Read the model definition and answer for the solid it produces. Units are mm, in the model's axes. Face numbers are marked on the shaded views. A direction names the side the tool comes from. Round coordinates to 2 decimals unless told otherwise and drop trailing zeros. Order: outer loops, then holes, each group sorted by start corner. A loop starts at its lowest first (then second) coordinate and runs counter-clockwise, first axis right, second up. Notation, with made-up numbers: M -35.75,26.25 L 20.25,26.25 A26 cw 20.25,57.25 Z; hole C 85.5,51.5 d7. An arc over 180 degrees is marked long. Answer as CSV lines item,"result".
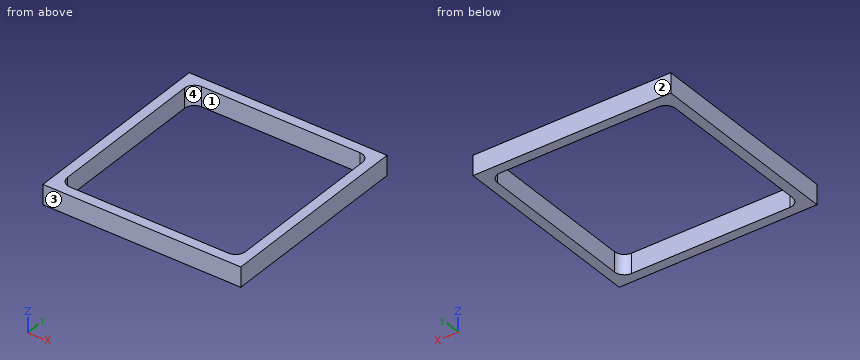
```python
from build123d import *

# Parameters (mm, degrees)
SKETCH1_W           = 127
SKETCH1_H           = 127
SKETCH1_W_2         = 114.3
SKETCH1_H_2         = 114.3
BOSS_EXTRUDE1_DEPTH = 12.7
FILLET1_R           = 6.35


with BuildPart() as part:
    # Sketch1 → Boss-Extrude1 (new body)
    with BuildSketch(Plane.XY):
        Rectangle(SKETCH1_W, SKETCH1_H)
        Rectangle(SKETCH1_W_2, SKETCH1_H_2, mode=Mode.SUBTRACT)
    extrude(amount=-BOSS_EXTRUDE1_DEPTH)

    # Fillet1
    fillet1_edges = [part.edges().sort_by_distance(p)[0] for p in [
        (57.15, 57.15, -6.35),
        (57.15, -57.15, -6.35),
        (-57.15, -57.15, -6.35),
        (-57.15, 57.15, -6.35),
    ]]
    fillet(fillet1_edges, radius=FILLET1_R)


solid = part.part
```
Item 1: A cutting plane is placed at B-B, the plane z = -9. Determine the outline of the cut face in (x, y).
Ans:
outline,"M -63.5,-63.5 L 63.5,-63.5 L 63.5,63.5 L -63.5,63.5 Z; hole M -57.15,-50.8 A6.35 ccw -50.8,-57.15 L 50.8,-57.15 A6.35 ccw 57.15,-50.8 L 57.15,50.8 A6.35 ccw 50.8,57.15 L -50.8,57.15 A6.35 ccw -57.15,50.8 Z"
Item 2: Determine the mould class of the marked faces 3 and 4 for opening direction X: +X half, -X half, draft (parallel to the pull), parting line (faces both ways), or undercut.
Ans:
face 3,"draft"
face 4,"undercut"
Item 3: A cutting plane is placed at A-A, the plane y = -47.5. Determine the outline of the cut face in (x, z).
Ans:
outline,"M -63.5,-12.7 L -57.15,-12.7 L -57.15,0 L -63.5,0 Z; M 57.15,-12.7 L 63.5,-12.7 L 63.5,0 L 57.15,0 Z"
Item 4: A tool of negligible diameter and unlimited length cuts with its end or side. For the marked faces 1 and 2, from which of +Z, -Z, +X, -X, +Y, -Y can it reach the whole face along a straight path? Write none if from no direction.
Ans:
face 1,"+Z, -Z"
face 2,"+Z, -Z, +X, -X, +Y"
Item 5: Find the intervals of material crossed by probe 1 along X at (y, z) = (-5.5, -4.25); probe 2 along Y at (x, z) = (55.5, -9), in increasing order. Write a range as [from, to].
Ans:
probe 1,"[-63.5, -57.15], [57.15, 63.5]"
probe 2,"[-63.5, -55.07], [55.07, 63.5]"
